Geometry check sheet. Reference: the model listing, model coordinates, mm. A direction names the side the tool comes from. Round coordinates to 2 decimals unless told otherwise and drop trailing zeros. Write each loop counter-clockwise with the first axis right and the second up, starting at its lowest first coordinate (ties: lowest second). Pieces come first, ordered by that corner, then holes. Notation, with made-up numbers: (28.25, 73) -> (48.25, 73) arc R17 ccw to (48.25, 92) -> close; hole circle Ø8 at (62.25, -27). An arc over 180 degrees is marked (long way). One line per question, with ' | ' between items.
```python
from build123d import *

# Parameters (mm, degrees)
BOSS_EXTRUDE1_DEPTH     = 30
CUT_EXTRUDE1_DEPTH      = 74.484692283
CUT_EXTRUDE1_DEPTH_BACK = 74.484692283
SKETCH3_R               = 7.5
CUT_EXTRUDE2_DEPTH      = 91
CUT_EXTRUDE2_DEPTH_BACK = 91
SKETCH5_R               = 15
CUT_EXTRUDE3_DEPTH      = 8
CUT_EXTRUDE4_REACH      = 86.876
SKETCH6_R               = 9
CUT_EXTRUDE5_DEPTH      = 74.484692283
CUT_EXTRUDE5_DEPTH_BACK = 74.484692283
SKETCH7_W               = 45
SKETCH7_H               = 25
SKETCH8_R               = 15
CUT_EXTRUDE6_DEPTH      = 8
CUT_EXTRUDE7_REACH      = 86.876
SKETCH9_R               = 9


with BuildPart() as part:
    # Sketch1 → Boss-Extrude1 (new, symmetric)
    with BuildSketch(Plane.XY):
        with BuildLine():
            Line((-60, 12.5), (-60, 30))
            Line((-60, 30), (30, 30))
            ThreePointArc((30, 30), (60, 0), (30, -30))
            Line((30, -30), (-60, -30))
            Line((-60, -30), (-60, -12.5))
            Line((-60, -12.5), (-15, -12.5))
            Line((-15, -12.5), (-15, 12.5))
            Line((-15, 12.5), (-60, 12.5))
        make_face()
    extrude(amount=BOSS_EXTRUDE1_DEPTH, both=True)

    # Sketch3 → Cut-Extrude1 (cut, two sides: drawn at the far end of the back side and taken through both)
    with BuildSketch(Plane.XY.offset(-CUT_EXTRUDE1_DEPTH_BACK)):
        Circle(SKETCH3_R)
    extrude(amount=CUT_EXTRUDE1_DEPTH + CUT_EXTRUDE1_DEPTH_BACK, mode=Mode.SUBTRACT)

    # Sketch4 → Cut-Extrude2 (cut, two sides: drawn at the far end of the back side and taken through both)
    with BuildSketch(Plane(origin=(0, 30, 0), x_dir=(1, 0, 0), z_dir=(0, 1, 0)).offset(-CUT_EXTRUDE2_DEPTH_BACK)):
        with BuildLine():
            Line((-30, 30), (-30, 42.770577687))
            Line((-30, 42.770577687), (-70.432292605, 42.770577687))
            Line((-70.432292605, 42.770577687), (-70.432292605, -35.727348426))
            Line((-70.432292605, -35.727348426), (-30, -35.727348426))
            Line((-30, -35.727348426), (-30, -30))
            ThreePointArc((-30, -30), (-60, 0), (-30, 30))
        make_face()
    extrude(amount=CUT_EXTRUDE2_DEPTH + CUT_EXTRUDE2_DEPTH_BACK, mode=Mode.SUBTRACT)

    # Sketch5 → Cut-Extrude3 (cut)
    with BuildSketch(Plane(origin=(0, 30, 0), x_dir=(1, 0, 0), z_dir=(0, 1, 0))):
        with Locations(Location((-30, 0, 0), (0, 0, 270))):
            Circle(SKETCH5_R)
    cut_extrude3 = extrude(amount=-CUT_EXTRUDE3_DEPTH, mode=Mode.SUBTRACT)

    # Sketch6 → Cut-Extrude4 (cut, up to next)
    with BuildSketch(Plane(origin=(0, 22, 0), x_dir=(1, 0, 0), z_dir=(0, 1, 0)), mode=Mode.PRIVATE) as cut_extrude4_sk1:
        with Locations(Location((-30, 0, 0), (0, 0, 270))):
            Circle(SKETCH6_R)
    cut_extrude4_tool1 = extrude(cut_extrude4_sk1.sketch, amount=-CUT_EXTRUDE4_REACH, mode=Mode.PRIVATE) & part.part
    cut_extrude4 = cut_extrude4_tool1.solids().sort_by_distance((-30, 22, 0))[0]
    add(cut_extrude4, mode=Mode.SUBTRACT)

    # Mirror1: Cut-Extrude3, Cut-Extrude4 across plane
    add(cut_extrude3.mirror(Plane.ZX), mode=Mode.SUBTRACT)
    add(cut_extrude4.mirror(Plane.ZX), mode=Mode.SUBTRACT)

    # Sketch7 → Cut-Extrude5 (cut, two sides: drawn at the far end of the back side and taken through both)
    with BuildSketch(Plane(origin=(0, 0, 0), x_dir=(1, 0, 0), z_dir=(0, 1, 0)).offset(-CUT_EXTRUDE5_DEPTH_BACK)):
        with Locations((37.5, 0)):
            Rectangle(SKETCH7_W, SKETCH7_H)
    extrude(amount=CUT_EXTRUDE5_DEPTH + CUT_EXTRUDE5_DEPTH_BACK, mode=Mode.SUBTRACT)

    # Sketch8 → Cut-Extrude6 (cut)
    with BuildSketch(Plane.XY.offset(30)):
        with Locations((30, 0)):
            Circle(SKETCH8_R)
    cut_extrude6 = extrude(amount=-CUT_EXTRUDE6_DEPTH, mode=Mode.SUBTRACT)

    # Sketch9 → Cut-Extrude7 (cut, up to next)
    with BuildSketch(Plane.XY.offset(22), mode=Mode.PRIVATE) as cut_extrude7_sk1:
        with Locations((30, 0)):
            Circle(SKETCH9_R)
    cut_extrude7_tool1 = extrude(cut_extrude7_sk1.sketch, amount=-CUT_EXTRUDE7_REACH, mode=Mode.PRIVATE) & part.part
    cut_extrude7 = cut_extrude7_tool1.solids().sort_by_distance((30, 0, 22))[0]
    add(cut_extrude7, mode=Mode.SUBTRACT)

    # Mirror2: Cut-Extrude6, Cut-Extrude7 across plane
    add(cut_extrude6.mirror(Plane.XY), mode=Mode.SUBTRACT)
    add(cut_extrude7.mirror(Plane.XY), mode=Mode.SUBTRACT)


solid = part.part
```
(1) Material ranges on line 1 (Z direction, x = 46.5, y = 19); line 2 (Y direction, x = -44.5, z = -2); line 3 (Y direction, x = 30, z = 25), recorded low to high.
Resolved:
line 1: z = -30 to -12.5, 12.5 to 30 | line 2: y = -22 to -12.5, 12.5 to 22 | line 3: y = -30 to -15, 15 to 30
(2) Sectioned sample at D-D on x = 32. Record the cut outline in (y, z).
Resolved:
outline: (-29.93, -30) -> (-14.87, -30) -> (-14.87, -22) -> (-8.77, -22) -> (-8.77, -12.5) -> (-29.93, -12.5) -> close; (-29.93, 12.5) -> (-8.77, 12.5) -> (-8.77, 22) -> (-14.87, 22) -> (-14.87, 30) -> (-29.93, 30) -> close; (8.77, -22) -> (14.87, -22) -> (14.87, -30) -> (29.93, -30) -> (29.93, -12.5) -> (8.77, -12.5) -> close; (8.77, 12.5) -> (29.93, 12.5) -> (29.93, 30) -> (14.87, 30) -> (14.87, 22) -> (8.77, 22) -> close
(3) Sectioned sample at A-A on x = 0. Record the cut outline in (y, z), then the cut area to 3 significant figures.
Resolved:
outline: (-30, -30) -> (-7.5, -30) -> (-7.5, 30) -> (-30, 30) -> close; (7.5, -30) -> (30, -30) -> (30, 30) -> (7.5, 30) -> close | area: 2,700 mm2
(4) Draft check along Z on faces 5 (the cylindrical face through (59.993, 0.66, 21.373)), 6 (the cylindrical face through (-59.993, -21.373, 0.66)), 7 (the cylindrical face through (-21.077, 17.316, -1.172)). Enter one of: +Z half, -Z half, draft (parallel to the pull), parting line (faces both ways), or undercut.
Resolved:
face 5: draft | face 6: parting line | face 7: undercut
(5) Sectioned sample at C-C on y = 0. Record the cut outline in (x, z), then the cut area to 3 significant figures.
Resolved:
outline: (-15, -30) -> (-7.5, -30) -> (-7.5, 30) -> (-15, 30) -> close; (7.5, -30) -> (15, -30) -> (15, -22) -> (21, -22) -> (21, -12.5) -> (15, -12.5) -> (15, 12.5) -> (21, 12.5) -> (21, 22) -> (15, 22) -> (15, 30) -> (7.5, 30) -> close; (39, -22) -> (45, -22) -> (45, -30) -> (60, -30) -> (60, -12.5) -> (39, -12.5) -> close; (39, 12.5) -> (60, 12.5) -> (60, 30) -> (45, 30) -> (45, 22) -> (39, 22) -> close | area: 1,650 mm2
(6) Sectioned sample at B-B on z = 0. Record the cut outline in (x, y), then the cut area to 3 significant figures.
Resolved:
outline: (-60, -30) -> (-45, -30) -> (-45, -22) -> (-39, -22) -> (-39, -12.5) -> (-60, -12.5) -> close; (-60, 12.5) -> (-39, 12.5) -> (-39, 22) -> (-45, 22) -> (-45, 30) -> (-60, 30) -> close; (-21, -22) -> (-15, -22) -> (-15, -30) -> (15, -30) -> (15, 30) -> (-15, 30) -> (-15, 22) -> (-21, 22) -> (-21, 12.5) -> (-15, 12.5) -> (-15, -12.5) -> (-21, -12.5) -> close; hole circle Ø15 at (0, 0) | area: 2,380 mm2
(7) Access from +Z, -Z, +X, -X, +Y, -Y to the whole of each face (thin tool, end or side, straight path). Record for faces 1 (the flat face through (-37, 12.5, -6)), 2 (the flat face through (37, 6, -12.5)), 3 (the cylindrical face through (-44.643, -26.056, -3.252)), 4 (the cylindrical face through (15.015, 0.66, 26.056)).
Resolved:
face 1: +Z, -Z, -X | face 2: +X, +Y, -Y | face 3: -Y | face 4: +Z
(8) Go/stop test with flat-tipped pins: pin 1 (2 mm diameter, centred on y = -15.5, z = 14, fed in from -X); pin 2 (8 mm diameter, centred on y = 5.5, z = -23.5, fed in from +X); pin 3 (1 mm diameter, centred on y = 10.5, z = -0.5, fed in from +X). Record where each tip stops, or that it passes through.
Resolved:
pin 1: stops at x = -57.04 | pin 2: stops at x = 59.96 | pin 3: stops at x = 15
